```python
from build123d import *

# Parameters (mm, degrees)
CROQUIS1_W              = 17
CROQUIS1_H              = 15
SALIENTE_EXTRUIR1_DEPTH = 20
CROQUIS2_R              = 2.75
CORTAR_EXTRUIR1_DEPTH   = 20
CROQUIS4_R              = 1.5
CORTAR_EXTRUIR3_DEPTH   = 20
CROQUIS7_W              = 8
CROQUIS7_H              = 3.948353597
CORTAR_EXTRUIR5_DEPTH   = 35
CROQUIS8_W              = 17
CROQUIS8_H              = 3
SALIENTE_EXTRUIR2_DEPTH = 15
CROQUIS9_W              = 15
CROQUIS9_H              = 3
SALIENTE_EXTRUIR3_DEPTH = 15
CROQUIS10_R             = 1.5
CORTAR_EXTRUIR6_DEPTH   = 10


with BuildPart() as part:
    # Croquis1 → Saliente-Extruir1 (new body)
    with BuildSketch(Plane(origin=(0, 0, 0), x_dir=(1, 0, 0), z_dir=(0, 1, 0))):
        Rectangle(CROQUIS1_W, CROQUIS1_H)
    extrude(amount=SALIENTE_EXTRUIR1_DEPTH)

    # Croquis2 → Cortar-Extruir1 (cut)
    with BuildSketch(Plane(origin=(0, 0, -7.5), x_dir=(-1, 0, 0), z_dir=(0, 0, -1))):
        with Locations((0, 7.5)):
            Circle(CROQUIS2_R)
        with BuildLine():
            Line((0.5, 20), (-0.5, 20))
            Line((-0.5, 20), (-0.5, 10.204163457))
            ThreePointArc((-0.5, 10.204163457), (0, 10.25), (0.5, 10.204163457))
            Line((0.5, 10.204163457), (0.5, 20))
        make_face()
    extrude(amount=-CORTAR_EXTRUIR1_DEPTH, mode=Mode.SUBTRACT)

    # Croquis4 → Cortar-Extruir3 (cut)
    with BuildSketch(Plane.ZY.offset(8.5)):
        with Locations((-0.5, 7.5)):
            Circle(CROQUIS4_R)
    extrude(amount=-CORTAR_EXTRUIR3_DEPTH, mode=Mode.SUBTRACT)

    # Croquis7 → Cortar-Extruir5 (cut)
    with BuildSketch(Plane.XY.offset(7.5)):
        with Locations((4.5, 18.025823201)):
            Rectangle(CROQUIS7_W, CROQUIS7_H)
        with Locations((-4.5, 18.025823201)):
            Rectangle(CROQUIS7_W, CROQUIS7_H)
    extrude(amount=-CORTAR_EXTRUIR5_DEPTH, mode=Mode.SUBTRACT)

    # Croquis8 → Saliente-Extruir2 (add)
    with BuildSketch(Plane.XY.offset(7.5)):
        with Locations((0, 1.5)):
            Rectangle(CROQUIS8_W, CROQUIS8_H)
    extrude(amount=SALIENTE_EXTRUIR2_DEPTH)

    # Croquis9 → Saliente-Extruir3 (add)
    with BuildSketch(Plane.ZY.offset(8.5)):
        with Locations((0, 1.5)):
            Rectangle(CROQUIS9_W, CROQUIS9_H)
    extrude(amount=SALIENTE_EXTRUIR3_DEPTH)

    # Croquis10 → Cortar-Extruir6 (cut)
    with BuildSketch(Plane.XZ):
        with Locations((-18.5, -3.5)):
            Circle(CROQUIS10_R)
        with Locations((-4.5, 17.5)):
            Circle(CROQUIS10_R)
        with Locations((4.5, 17.5)):
            Circle(CROQUIS10_R)
        with Locations((-18.5, 3.5)):
            Circle(CROQUIS10_R)
    extrude(amount=-CORTAR_EXTRUIR6_DEPTH, mode=Mode.SUBTRACT)


solid = part.part
```
Check sheet for the modelled part. Datum: model origin and axes. Units: mm. A direction names the side the tool comes from. Give positions to 0.01 mm unless a question says otherwise; leave off trailing zeros. Write each loop counter-clockwise with the first axis right and the second up, starting at its lowest first coordinate (ties: lowest second). Pieces come first, ordered by that corner, then holes. Notation, with made-up numbers: (74.25, 0.25) - (86.25, 0.25) arc R21 cw to (86.25, 29.25) - close; hole circle Ø3 at (6, 8). An arc over 180 degrees is marked (long way). Answer as a JSON object with one key per item and string values. Group by question number.
1) Access from +Z, -Z, +X, -X, +Y, -Y to the whole of each face (thin tool, end or side, straight path). Record for faces 1 (the face through (-23.5, 2, 0)), 2 (the face through (0, 3, 15)), 3 (the face through (-0.5, 13, 0)).
2) Sectioned sample at D-D (y = 14). Record the cut outline in (x, z).
3) Depth check by flat-ended pin: P1, Ø4.5, axis at x = -4, z = 17, coming from the +Y side; P2, Ø2.5, axis at x = -4.5, z = 17.5, coming from the -Y side; P3, Ø0.9, axis at x = -15.5, y = 1.5, coming from the +Z side; P4, Ø3, axis at y = 12, z = 0, coming from the -X side. Enter the tip coordinate at first touch or a pass-through.
4) Sectioned sample at B-B (z = -3.5). Record the cut outline in (x, y).
5) Sectioned sample at C-C (y = 7.5). Record the cut outline in (x, z), then the cut area to 3 significant figures.
6) Release check for a two-part mould opening along X. For faces 4 (the face through (0.114, 4.752, -0.105)), 5 (the face through (4.305, 1.479, 18.987)), 6 (the face through (-8.5, 1, 15)), 7 (the face through (-16, 3, 0)) record: pulls with the +X half, pulls with the -X half, needs draft (parallel to the pull), parting line crosses it, or undercut.
7) Thickness scan on probe 1 along Z at (x, y) = (-18.5, 0.65); probe 2 along Z at (x, y) = (4.5, 1.25); probe 3 along X at (y, z) = (6, -2). Record the ranges inside material, lowest first. Write a range as from..to.
8) Sectioned sample at A-A (x = 4.5). Record the cut outline in (y, z).
Geometry results:
{
 "1": {"face 1": "+Z, -Z, -X, +Y, -Y", "face 2": "+Z, +X, -X, +Y", "face 3": "+Z, -Z, +Y"},
 "2": {"outline": "(-8.5, -7.5) - (-0.5, -7.5) - (-0.5, 7.5) - (-8.5, 7.5) - close; (0.5, -7.5) - (8.5, -7.5) - (8.5, 7.5) - (0.5, 7.5) - close"},
 "3": {"P1": "stops at y = 3", "P2": "passes through", "P3": "stops at z = 7.5", "P4": "stops at x = -8.5"},
 "4": {"outline": "(-23.5, 0) - (-20, 0) - (-20, 3) - (-23.5, 3) - close; (-17, 0) - (8.5, 0) - (8.5, 16.05) - (0.5, 16.05) - (0.5, 10.2) arc R2.75 cw (long way) to (-0.5, 10.2) - (-0.5, 16.05) - (-8.5, 16.05) - (-8.5, 3) - (-17, 3) - close"},
 "5": {"outline": "(-8.5, -7.5) - (-2.75, -7.5) - (-2.75, -2) - (-8.5, -2) - close; (-8.5, 1) - (-2.75, 1) - (-2.75, 7.5) - (-8.5, 7.5) - close; (2.75, -7.5) - (8.5, -7.5) - (8.5, -2) - (2.75, -2) - close; (2.75, 1) - (8.5, 1) - (8.5, 7.5) - (2.75, 7.5) - close", "area": "138 mm^2"},
 "6": {"face 4": "undercut", "face 5": "undercut", "face 6": "pulls with the -X half", "face 7": "needs draft"},
 "7": {"probe 1": "z = -7.5..-5, -2..2, 5..7.5", "probe 2": "z = -7.5..16, 19..22.5", "probe 3": "x = -8.5..-2.3, 2.3..8.5"},
 "8": {"outline": "(0, -7.5) - (16.05, -7.5) - (16.05, 7.5) - (3, 7.5) - (3, 16) - (0, 16) - close; (0, 19) - (3, 19) - (3, 22.5) - (0, 22.5) - close; hole circle Ø3 at (7.5, -0.5)"}
}
